Answer from the drawing. Dimensions are ordinates in mm from the lowest x, y and z of the part. A direction names the side the tool comes from. Give positions to 0.01 mm unless a question says otherwise; leave off trailing zeros. Loops run counter-clockwise (first coordinate to the right, second up) from the corner with the lowest first, then second, coordinate; pieces in that order, holes last.
(1) Find section D-D, the plane z = 6. Write down the section's boundary in (x, y).
(2) Find section A-A, the plane y = 18. Write down the section's boundary in (x, z), then the cut area to 3 significant figures.
(3) Which of the six approach directions +Z, -Z, +X, -X, +Y, -Y give full straight-line access (tool end or side, diameter ignored) to the marked faces 5, 6, 7, 8 and 9?
(4) Find section C-C, the plane y = 10.75. Write down the section's boundary in (x, z).
(5) Straight lines are drawn through the part: probe 1 along X at (y, z) = (16.5, 35.5); probe 2 along X at (y, z) = (11, 30.5); probe 3 along Z at (x, y) = (16.5, 15). For each, find the intervals that lie inside material, in ascending order.
(6) Determine the mould class of the marked faces 1, 2, 3 and 4 for opening direction X: pulls with the +X half, pulls with the -X half, needs draft (parallel to the pull), parting line crosses it, or undercut.
(7) Find section B-B, the plane z = 18. Write down the section's boundary in (x, y).
(8) Each of these flat-tipped pins is pushed along its axis until it touches: P1, Ø8, axis at y = 18.5, z = 38.5, coming from the -X side; P2, Ø1, axis at y = 7, z = 26, coming from the +X side; P3, Ø6, axis at x = 40.5, z = 42, coming from the -Y side; P4, Ø4, axis at x = 18, y = 18, coming from the +Z side. Where does it stop, or does it pass through?
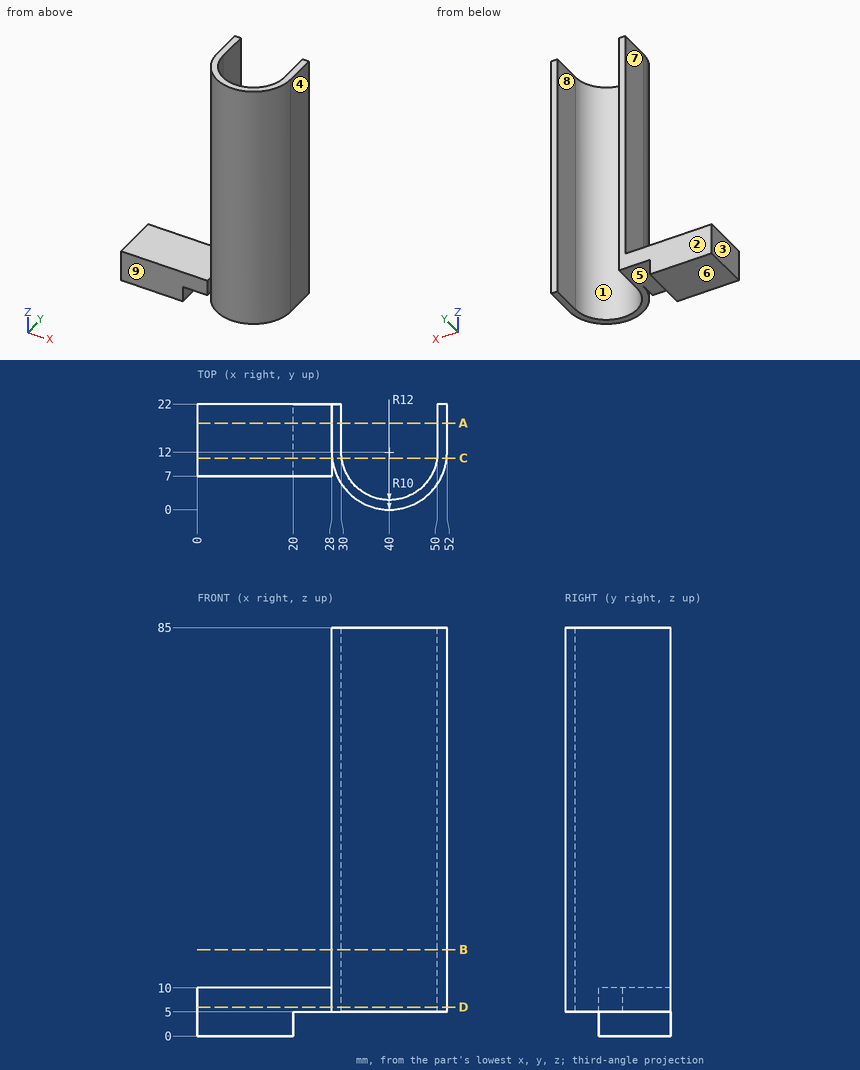
Entries:
1. outline: (0, 7) - (28, 7) - (28, 12) arc R12 ccw to (52, 12) - (52, 22) - (50, 22) - (50, 12) arc R10 cw to (30, 12) - (30, 22) - (0, 22) - close
2. outline: (0, 0) - (20, 0) - (20, 5) - (30, 5) - (30, 85) - (28, 85) - (28, 10) - (0, 10) - close; (50, 5) - (52, 5) - (52, 85) - (50, 85) - close
2. area: 560 mm2
3. face 5: -Z, +X, +Y, -Y
3. face 6: -Z, +X, -X, +Y, -Y
3. face 7: +Z, -X, +Y, -Y
3. face 8: +Z, -Z, +Y
3. face 9: +Z, -Z, -X, -Y
4. outline: (0, 0) - (20, 0) - (20, 5) - (28, 5) - (28, 10) - (0, 10) - close; (28.07, 5) - (30.08, 5) - (30.08, 85) - (28.07, 85) - close; (49.92, 5) - (51.93, 5) - (51.93, 85) - (49.92, 85) - close
5. probe 1: x = 28 to 30, 50 to 52
5. probe 2: x = 28.04 to 30.05, 49.95 to 51.96
5. probe 3: z = 0 to 10
6. face 1: undercut
6. face 2: needs draft
6. face 3: pulls with the -X half
6. face 4: pulls with the +X half
7. outline: (28, 12) arc R12 ccw to (52, 12) - (52, 22) - (50, 22) - (50, 12) arc R10 cw to (30, 12) - (30, 22) - (28, 22) - close
8. P1: stops at x = 28
8. P2: stops at x = 51.12
8. P3: stops at y = 0
8. P4: stops at z = 10
